The listing builds one solid part. Answer for the finished solid, in the listing's coordinates (mm). Coordinates: 2 decimals unless noted, no trailing zeros. Order: outer loops, then holes, each group sorted by start corner. A loop starts at its lowest first (then second) coordinate and runs counter-clockwise, first axis right, second up.
from build123d import *

# Parameters (mm, degrees)
BOSS_EXTRU_1_DEPTH      = 3
ESQUISSE2_R             = 1.1
ENL_V_MAT_EXTRU_1_DEPTH = 3
ESQUISSE3_R             = 1.1
ENL_V_MAT_EXTRU_2_DEPTH = 3
CONG_1_R                = 3
CONG_1_OF_SYM_TRIE1_R   = 3


with BuildPart() as part:
    # Esquisse1 → Boss.-Extru.1 (new body)
    with BuildSketch(Plane.XY):
        Polygon((-13.5, 5), (-49, 5), (-49, 0), (-49, -7), (-43, -7), (-43, 0), (0, 0), (0, 5), (-7.5, 5), (-7.5, 30), (-13.5, 30), align=None)
    boss_extru_1 = extrude(amount=BOSS_EXTRU_1_DEPTH)

    # Esquisse2 → Enlèv. mat.-Extru.1 (cut)
    with BuildSketch(Plane.XY.offset(3)):
        with Locations((-45.5, -3.5)):
            Circle(ESQUISSE2_R)
    enl_v_mat_extru_1 = extrude(amount=-ENL_V_MAT_EXTRU_1_DEPTH, mode=Mode.SUBTRACT)

    # Esquisse3 → Enlèv. mat.-Extru.2 (cut)
    with BuildSketch(Plane.XY.offset(3)):
        with Locations((-10.5, 15)):
            Circle(ESQUISSE3_R)
        with Locations((-10.5, 27.5)):
            Circle(ESQUISSE3_R)
    enl_v_mat_extru_2 = extrude(amount=-ENL_V_MAT_EXTRU_2_DEPTH, mode=Mode.SUBTRACT)

    # Congé1
    cong_1_edges = [part.edges().sort_by_distance(p)[0] for p in [
        (-13.5, 5, 1.5),
        (-7.5, 5, 1.5),
        (-7.5, 30, 1.5),
        (-13.5, 30, 1.5),
        (-49, 5, 1.5),
        (-49, -7, 1.5),
    ]]
    fillet(cong_1_edges, radius=CONG_1_R - 0.0001)  # a hair under: the kernel refuses the full size

    # Symétrie1: Boss.-Extru.1, Enlèv. mat.-Extru.1, Enlèv. mat.-Extru.2 across plane
    add(boss_extru_1.mirror(Plane(origin=(0, 0, 0), x_dir=(0, 0, 1), z_dir=(1, 0, 0))))
    add(enl_v_mat_extru_1.mirror(Plane(origin=(0, 0, 0), x_dir=(0, 0, 1), z_dir=(1, 0, 0))), mode=Mode.SUBTRACT)
    add(enl_v_mat_extru_2.mirror(Plane(origin=(0, 0, 0), x_dir=(0, 0, 1), z_dir=(1, 0, 0))), mode=Mode.SUBTRACT)

    # Congé1 of Symétrie1
    cong_1_of_sym_trie1_edges = [part.edges().sort_by_distance(p)[0] for p in [
        (13.5, 5, 1.5),
        (7.5, 5, 1.5),
        (7.5, 30, 1.5),
        (13.5, 30, 1.5),
        (49, 5, 1.5),
        (49, -7, 1.5),
    ]]
    fillet(cong_1_of_sym_trie1_edges, radius=CONG_1_OF_SYM_TRIE1_R - 0.0001)  # a hair under: the kernel refuses the full size


solid = part.part
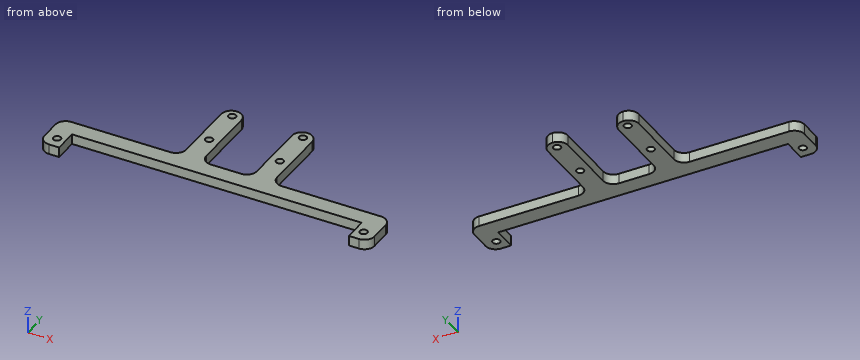
1) Section A-A (z = 0.65) is taken. Give the number of separate pieces and of enclosed holes in the cut face, then the cut area to 3 significant figures.
2) Consider L1, parallel to Y at x = 10.5, z = 2.15; L2, parallel to X at y = 19.5, z = 2.1; L3, parallel to Y at x = -45.5, z = 1.3. Determine where each line is inside the solid, lowest interval first.
3) Section B-B (y = 15) is taken. Give the vertices of the cut face in (x, z).
4) Section D-D (x = 6) is taken. Give the vertices of the cut face in (y, z).
5) Section C-C (x = -22) is taken. Give the vertices of the cut face in (y, z).
6) Each of these flat-tipped pins is pushed along its axis until it touches: P1, Ø1.5, axis at y = 19.5, z = 1.5, coming from the +X side; P2, Ø0.9, axis at x = 6, z = 1, coming from the -Y side; P3, Ø1.5, axis at y = 19, z = 2, coming from the -X side; P4, Ø1.8, axis at x = 45.5, y = -3.5, coming from the -Z side. Where does it stop, or does it pass through?
Filled sheet:
1. separate pieces: 1
1. enclosed holes: 6
1. area: 843 mm2
2. L1: y = 0 to 13.9, 16.1 to 26.4, 28.6 to 30
2. L2: x = -13.5 to -7.5, 7.5 to 13.5
2. L3: y = -7 to -4.6, -2.4 to 5
3. outline: (-13.5, 0) - (-11.6, 0) - (-11.6, 3) - (-13.5, 3) - close; (-9.4, 0) - (-7.5, 0) - (-7.5, 3) - (-9.4, 3) - close; (7.5, 0) - (9.4, 0) - (9.4, 3) - (7.5, 3) - close; (11.6, 0) - (13.5, 0) - (13.5, 3) - (11.6, 3) - close
4. outline: (0, 0) - (5.4, 0) - (5.4, 3) - (0, 3) - close
5. outline: (0, 0) - (5, 0) - (5, 3) - (0, 3) - close
6. P1: stops at x = 13.5
6. P2: stops at y = 0
6. P3: stops at x = -13.5
6. P4: passes through
